Drawing for the job (mm, zero at the part's lowest x, y, z). A direction names the side the tool comes from. Give positions to 0.01 mm unless a question says otherwise; leave off trailing zeros. Order: outer loops, then holes, each group sorted by start corner. A loop starts at its lowest first (then second) coordinate and runs counter-clockwise, first axis right, second up. Notation, with made-up numbers: (-23.75, 11.25) - (-4.75, 11.25) arc R27 cw to (-4.75, 35.25) - close; hole circle Ø6 at (38.25, 33). An arc over 180 degrees is marked (long way). Write each question's results on one line, items separated by ' | '. Start each with the question number.
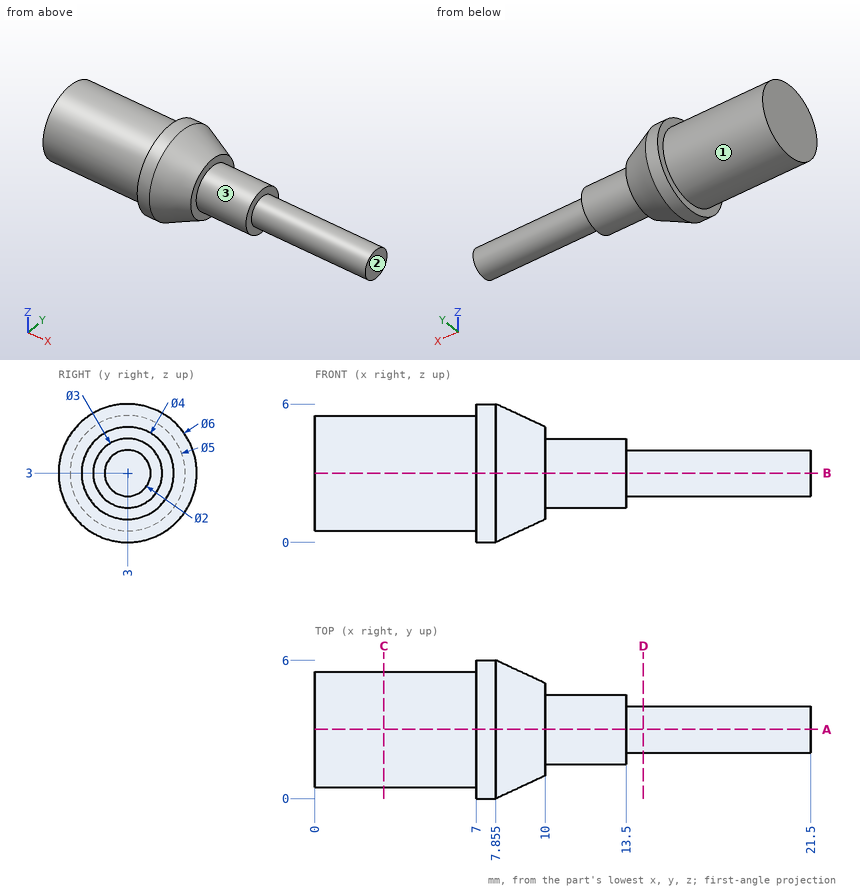
Item 1: Cut at C-C, the plane x = 3. List the corners of the cut face in (y, z).
Item 2: Cut at D-D, the plane x = 14.25. List the corners of the cut face in (y, z).
Item 3: Probe line 1 along X through (y, z) = (3, 1.9); line 2 along X through (y, z) = (3.4, 1.35); line 3 along Z through (x, y) = (4, 3.1). List the from-to ranges inside material, lowest first. Write a range as from..to.
Item 4: Flat gauge pins, fed straight in: pin 1 Ø3 at (y, z) = (1.5, 2.5) entering from +X; pin 2 Ø1 at (x, y) = (13.5, 1.5) entering from -Z. Where does each tip first touch, or does it go through?
Item 5: Cut at A-A, the plane y = 3. List the corners of the cut face in (x, z) (1 decimal).
Item 6: Which spindle directions (+Z, -Z, +X, -X, +Y, -Y) get a long thin tool onto all of the face, cutting with end or side? Do the marked faces 1, 2 and 3. Say none if no direction does.
Values found:
1) outline: circle Ø5 at (3, 3)
2) outline: circle Ø2 at (3, 3)
3) line 1: x = 0..13.5 | line 2: x = 0..10 | line 3: z = 0.5..5.5
4) pin 1: stops at x = 21.5 | pin 2: stops at z = 1.88
5) outline: (0, 0.5) - (7, 0.5) - (7, 0) - (7.9, 0) - (10, 1) - (10, 1.5) - (13.5, 1.5) - (13.5, 2) - (21.5, 2) - (21.5, 4) - (13.5, 4) - (13.5, 4.5) - (10, 4.5) - (10, 5) - (7.9, 6) - (7, 6) - (7, 5.5) - (0, 5.5) - close
6) face 1: -X | face 2: +Z, -Z, +X, +Y, -Y | face 3: +X
